CAD build for the part. Positions are in the model's coordinates, mm. A direction names the side the tool comes from. Round coordinates to 2 decimals unless told otherwise and drop trailing zeros. Order: outer loops, then holes, each group sorted by start corner. A loop starts at its lowest first (then second) coordinate and runs counter-clockwise, first axis right, second up. Notation, with made-up numbers: M 27.25,43 L 79.25,43 A9 ccw 79.25,49 Z; hole C -24.5,22 d2. An arc over 180 degrees is marked long. Put each result on its own line as item: value.
```python
from build123d import *

# Parameters (mm, degrees)
SKETCH1_R           = 2.38125
BOSS_EXTRUDE1_DEPTH = 3.175


with BuildPart() as part:
    # Sketch1 → Boss-Extrude1 (new body)
    with BuildSketch(Plane.XY):
        with BuildLine():
            Line((330.2, 0), (-330.2, 0))
            Line((-330.2, 0), (-330.2, 203.2))
            Line((-330.2, 203.2), (-279.4, 203.2))
            Line((-279.4, 203.2), (-279.4, 152.4))
            ThreePointArc((-279.4, 152.4), (-264.521024484, 116.478975516), (-228.6, 101.6))
            Line((-228.6, 101.6), (228.6, 101.6))
            ThreePointArc((228.6, 101.6), (264.521024484, 116.478975516), (279.4, 152.4))
            Line((279.4, 152.4), (279.4, 203.2))
            Line((279.4, 203.2), (330.2, 203.2))
            Line((330.2, 203.2), (330.2, 0))
        make_face()
        with Locations((-304.8, 177.8)):
            Circle(SKETCH1_R, mode=Mode.SUBTRACT)
        with Locations((-304.8, 127)):
            Circle(SKETCH1_R, mode=Mode.SUBTRACT)
        with Locations((-304.8, 76.2)):
            Circle(SKETCH1_R, mode=Mode.SUBTRACT)
        with Locations((-304.8, 25.4)):
            Circle(SKETCH1_R, mode=Mode.SUBTRACT)
        with Locations((304.8, 177.8)):
            Circle(SKETCH1_R, mode=Mode.SUBTRACT)
        with Locations((304.8, 127)):
            Circle(SKETCH1_R, mode=Mode.SUBTRACT)
        with Locations((304.8, 76.2)):
            Circle(SKETCH1_R, mode=Mode.SUBTRACT)
        with Locations((304.8, 25.4)):
            Circle(SKETCH1_R, mode=Mode.SUBTRACT)
    extrude(amount=BOSS_EXTRUDE1_DEPTH)


solid = part.part
```
Item 1: Tool access for faces 3 (the cylindrical face through (-264.914, 116.876, 1.565)), 4 (the flat face through (5, 58, 0)): list every direction of +Z, -Z, +X, -X, +Y, -Y with a clear straight run to the whole face (end or side of a thin tool).
Answers below:
face 3: +Z, -Z, +Y
face 4: -Z, +X, -X, +Y, -Y
Item 2: Probe line 1 along Y through (x, z) = (304.8, 2); line 2 along X through (y, z) = (187.5, 0.8); line 3 along X through (y, z) = (149.5, 1.8). List the from-to ranges inside material, lowest first. Write a range as [from, to].
Answers below:
line 1: [0, 23.02], [27.78, 73.82], [78.58, 124.62], [129.38, 175.42], [180.18, 203.2]
line 2: [-330.2, -279.4], [279.4, 330.2]
line 3: [-330.2, -279.32], [279.32, 330.2]
Item 3: Band-saw the part on D-D on x = -259.5. Give the cut face in (y, z) (3 decimals).
Answers below:
outline: M 0,0 L 112.078,0 L 112.078,3.175 L 0,3.175 Z
Item 4: Pin check, flat tip, straight feed: P1, Ø6, axis at x = -250.5, y = 111, coming from the -Z side. Stop position of the tip, or through.
Answers below:
P1: through
Item 5: Band-saw the part on A-A on z = 0.8. State how many separate pieces and enclosed holes the cut face has, and give its area (3 significant figures).
Answers below:
separate pieces: 1
enclosed holes: 8
area: 78,400 mm²
Item 6: Mould opens along X. For faces 1 (the flat face through (5, 58, 3.175)), 2 (the cylindrical face through (264.124, 116.086, 1.565)) say: pulls with the +X half, pulls with the -X half, needs draft (parallel to the pull), parting line crosses it, or undercut.
Answers below:
face 1: needs draft
face 2: undercut
Item 7: Band-saw the part on B-B on y = 144. Give the cut face in (x, z) (3 decimals), and give its area (3 significant figures).
Answers below:
outline: M -330.2,0 L -278.701,0 L -278.701,3.175 L -330.2,3.175 Z; M 278.701,0 L 330.2,0 L 330.2,3.175 L 278.701,3.175 Z
area: 327 mm²
Item 8: Band-saw the part on C-C on x = 59.5. Give the cut face in (y, z) (3 decimals).
Answers below:
outline: M 0,0 L 101.6,0 L 101.6,3.175 L 0,3.175 Z
